For this review, take the finished solid that the model builds, in its own axes (mm). Give positions to 0.01 mm unless a question says otherwise; leave off trailing zeros. Order: outer loops, then holes, each group sorted by start corner. A loop starts at its lowest first (then second) coordinate and runs counter-clockwise, first axis right, second up.
Item 1: Consider section B-B (x = 30). Give the boundary of the cut face in (y, z).
Item 2: For P1, Ø1.8, axis at x = -71, y = -1, coming from the +Z side, flat-tipped, find the tip position at first contact; note if it passes through.
Item 3: For probe 1 along Y at (x, z) = (70, 5.25); probe 2 along Y at (x, z) = (72, 0.5); probe 3 along X at (y, z) = (-8.5, 8.5), list the stretches that pass through material, from the lowest coordinate up.
Item 4: Consider section A-A (z = 2.75). Give the number of separate pieces and of enclosed holes in the cut face, plus the area to 3 significant figures.
```python
from build123d import *

# Parameters (mm, degrees)
SKETCH1_W           = 160
SKETCH1_H           = 30
BOSS_EXTRUDE1_DEPTH = 10
SKETCH2_R           = 3
CUT_EXTRUDE1_DEPTH  = 9.8
FILLET2_R           = 10


with BuildPart() as part:
    # Sketch1 → Boss-Extrude1 (new body)
    with BuildSketch(Plane.XY):
        Rectangle(SKETCH1_W, SKETCH1_H)
    extrude(amount=BOSS_EXTRUDE1_DEPTH)

    # Sketch2 → Cut-Extrude1 (cut)
    with BuildSketch(Plane.XY.offset(10)):
        with Locations((30, 0)):
            Circle(SKETCH2_R)
        with Locations((-30, 0)):
            Circle(SKETCH2_R)
        with Locations((-70, 0)):
            Circle(SKETCH2_R)
        with Locations((-50, 0)):
            Circle(SKETCH2_R)
        with Locations((50, 0)):
            Circle(SKETCH2_R)
        with Locations((70, 0)):
            Circle(SKETCH2_R)
        with Locations((-10, 0)):
            Circle(SKETCH2_R)
        with Locations((10, 0)):
            Circle(SKETCH2_R)
    extrude(amount=-CUT_EXTRUDE1_DEPTH, mode=Mode.SUBTRACT)

    # Fillet2
    fillet2_edges = [part.edges().sort_by_distance(p)[0] for p in [
        (80, -15, 5),
        (-80, -15, 5),
        (-80, 15, 5),
        (80, 15, 5),
    ]]
    fillet(fillet2_edges, radius=FILLET2_R)


solid = part.part
```
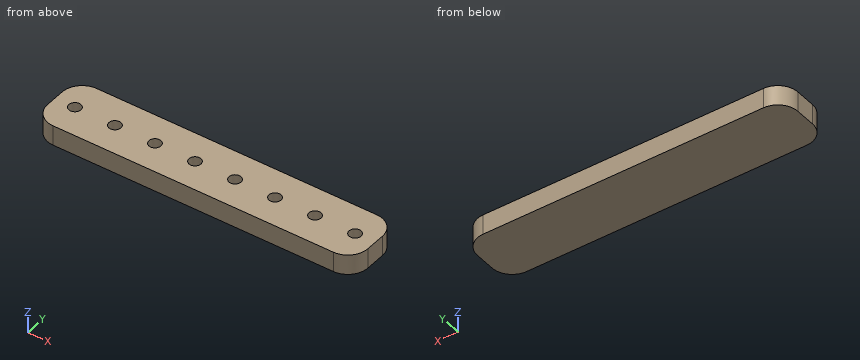
Resolved:
1. outline: (-15, 0) - (15, 0) - (15, 10) - (3, 10) - (3, 0.2) - (-3, 0.2) - (-3, 10) - (-15, 10) - close
2. P1: stops at z = 0.2
3. probe 1: y = -15 to -3, 3 to 15
3. probe 2: y = -14.8 to -2.24, 2.24 to 14.8
3. probe 3: x = -79.37 to 79.37
4. separate pieces: 1
4. enclosed holes: 8
4. area: 4,490 mm2
